from build123d import *

# Parameters (mm, degrees)
SKETCH_1_W          = 45
SKETCH_1_H          = 41
EXTRUDE_1_DEPTH     = 3
SKETCH_2_W          = 12
SKETCH_2_H          = 10
EXTRUDE_2_DEPTH     = 3
EXTRUDE_3_DEPTH     = 3
SKETCH_4_R          = 1.55
CUT_EXTRUDE_1_DEPTH = 3
FILLET_1_R          = 2


with BuildPart() as part:
    # 草图1 → 凸台-拉伸1 (new body)
    with BuildSketch(Plane.XY):
        Rectangle(SKETCH_1_W, SKETCH_1_H)
    extrude(amount=EXTRUDE_1_DEPTH)

    # 草图2 → 凸台-拉伸2 (add)
    with BuildSketch(Plane.XY.offset(3)):
        with Locations((22.5, 0)):
            Rectangle(SKETCH_2_W, SKETCH_2_H)
        with Locations((-22.5, 0)):
            Rectangle(SKETCH_2_W, SKETCH_2_H)
    extrude(amount=-EXTRUDE_2_DEPTH)

    # 草图3 → 凸台-拉伸3 (add)
    with BuildSketch(Plane.XY.offset(3)):
        Polygon((-22.5, 20.5), (-28.5, 5), (-22.5, 5), align=None)
        Polygon((22.5, 5), (22.5, 20.5), (28.5, 5), align=None)
        Polygon((-28.5, -5), (-22.5, -5), (-22.5, -20.5), align=None)
        Polygon((22.5, -20.5), (28.5, -5), (22.5, -5), align=None)
    extrude(amount=-EXTRUDE_3_DEPTH)

    # 草图4 → 切除-拉伸1 (cut)
    with BuildSketch(Plane.XY.offset(3)):
        with Locations((25.5, 0)):
            Circle(SKETCH_4_R)
        with Locations(Location((-25.5, 0, 0), (0, 0, 180))):
            Circle(SKETCH_4_R)
    extrude(amount=-CUT_EXTRUDE_1_DEPTH, mode=Mode.SUBTRACT)

    # 圆角1
    fillet_1_edges = [part.edges().sort_by_distance(p)[0] for p in [
        (28.5, -5, 1.5),
        (28.5, 5, 1.5),
        (-28.5, 5, 1.5),
        (-28.5, -5, 1.5),
        (22.5, -20.5, 1.5),
        (-22.5, -20.5, 1.5),
        (-22.5, 20.5, 1.5),
        (22.5, 20.5, 1.5),
    ]]
    fillet(fillet_1_edges, radius=FILLET_1_R)


solid = part.part
Verification items for the finished model (mm, model axes). Give positions to 0.01 mm unless a question says otherwise; leave off trailing zeros. Write each loop counter-clockwise with the first axis right and the second up, starting at its lowest first coordinate (ties: lowest second). Pieces come first, ordered by that corner, then holes. Notation, with made-up numbers: M 9.5,81 L 62.5,81 A5 ccw 62.5,85 Z; hole C 53.25,16.25 d5. An arc over 180 degrees is marked long. Write item = value, one per line.
(1) Sectioned sample at D-D (y = -15.5). Record the cut outline in (x, z).
Found:
outline = M -24.44,0 L 24.44,0 L 24.44,3 L -24.44,3 Z
(2) Material ranges on line 1 (X direction, y = 0.5, z = 0.2); line 2 (X direction, y = -9, z = 2.7); line 3 (X direction, y = 11, z = 1.9), recorded low to high.
Found:
line_1 = -28.5 to -26.97, -24.03 to 24.03, 26.97 to 28.5
line_2 = -26.95 to 26.95
line_3 = -26.18 to 26.18
(3) Sectioned sample at C-C (x = 25.5). Record the cut outline in (y, z), then the cut area to 3 significant figures.
Found:
outline = M -12.75,0 L -1.55,0 L -1.55,3 L -12.75,3 Z; M 1.55,0 L 12.75,0 L 12.75,3 L 1.55,3 Z
area = 67.2 mm2
(4) Sectioned sample at B-B (z = 2.4). Record the cut outline in (x, y), then the cut area to 3 significant figures.
Found:
outline = M -28.5,-4.63 A2 ccw -28.37,-5.35 L -22.99,-19.22 A2 ccw -21.13,-20.5 L 21.13,-20.5 A2 ccw 22.99,-19.22 L 28.37,-5.35 A2 ccw 28.5,-4.63 L 28.5,4.63 A2 ccw 28.37,5.35 L 22.99,19.22 A2 ccw 21.13,20.5 L -21.13,20.5 A2 ccw -22.99,19.22 L -28.37,5.35 A2 ccw -28.5,4.63 Z; hole C -25.5,0 d3.1; hole C 25.5,0 d3.1
area = 2,130 mm2
(5) Draft check along Y on faces 1 (the face through (-28.5, 0, 2)), 2 (the face through (-23.95, -0.07, 1.52)), 3 (the face through (26.932, -0.594, 1.521)), 4 (the face through (-25.642, 12.382, 1.521)). Enter one of: released by +Y, released by -Y, zero draft, split by the parting line, or undercut.
Found:
face_1 = zero draft
face_2 = undercut
face_3 = undercut
face_4 = released by +Y
(6) Sectioned sample at A-A (y = 0). Record the cut outline in (x, z), then the cut area to 3 significant figures.
Found:
outline = M -28.5,0 L -27.05,0 L -27.05,3 L -28.5,3 Z; M -23.95,0 L 23.95,0 L 23.95,3 L -23.95,3 Z; M 27.05,0 L 28.5,0 L 28.5,3 L 27.05,3 Z
area = 152 mm2
(7) Go/stop test with a flat-tipped pin: pin 1 Ø1.9 at (x, y) = (25.5, 0) entering from +Z. Record where the tip stops, or that it passes through.
Found:
pin_1 = through
